Source: CAD feature listing. Evaluate the final solid. Frame: model axes, mm. A direction names the side the tool comes from. Give positions to 0.01 mm unless a question says otherwise; leave off trailing zeros. Order: outer loops, then holes, each group sorted by start corner. A loop starts at its lowest first (then second) coordinate and runs counter-clockwise, first axis right, second up. Notation, with made-up numbers: (45.5, 18) - (54.5, 18) arc R26 ccw to (54.5, 32) - close; hole circle Ø4 at (45.5, -11.5). An arc over 180 degrees is marked (long way). One line per item, written item: value. Start each with the question number.
Autodesk Inventor part; units mm, degrees
ref_plane "YZ Plane" through (0, 0, 0) normal (1, 0, 0) x (0, 1, 0)
ref_plane "XZ Plane" through (0, 0, 0) normal (0, 1, 0) x (-1, 0, 0)
ref_plane "XY Plane" through (0, 0, 0) normal (0, 0, 1) x (1, 0, 0)
sketch "Sketch1" plane through (0, 0, 0) normal (0, 1, 0) x (-1, 0, 0)
  line L0 (0, 4.9984) -> (-15, 4.9984)
  line L1 (-15, 4.9984) -> (-15, -15.0016)
  line L2 (-15, -15.0016) -> (0, -15.0016)
  line L3 (0, -15.0016) -> (0, 4.9984)
  dimension "d0" = 15
  dimension "d1" = 20
extrude "Plate1" add sketch "Sketch1" along normal blind 0.5
sketch "Sketch2" plane through (0, 1.3536, -15.3552) normal (0, 0.7071068, -0.7071068) x (-1, 0, 0)
  line L0 (-15, 0) -> (0, 0)
  line L1 (0, 0) -> (0, 2.5858)
  line L2 (0, 2.5858) -> (-15, 2.5858)
  line L3 (-15, 2.5858) -> (-15, 0)
edge flange "Flange1" height 5 angle 135 thickness 0.5 bend radius 0.5 thickness toward (0, 0.7071068, -0.7071068) relief tear relief width 0.5 relief depth 0.25 edges at (7.5, 0.5, -15.0016) wall of the first edge with corners at (15, 1.3536, -15.3552) (0, 1.3536, -15.3552) (0, 3.182, -13.5267) (15, 3.182, -13.5267)
bend "Bend1"
corner "Corner1"
sketch "Sketch3" plane through (15, 3.8891, -13.7338) normal (0, 0, 1) x (1, 0, 0)
  line L0 (-15, 0) -> (0, 0)
  line L1 (0, 0) -> (0, 26.5858)
  line L2 (0, 26.5858) -> (-15, 26.5858)
  line L3 (-15, 26.5858) -> (-15, 0)
edge flange "Flange2" height 27 angle 45 thickness 0.5 bend radius 0.5 thickness toward (0, 0, 1) relief tear relief width 0.5 relief depth 0.25 edges at (7.5, 3.5355, -13.8803) wall of the first edge with corners at (0, 3.8891, -13.7338) (15, 3.8891, -13.7338) (15, 30.4749, -13.7338) (0, 30.4749, -13.7338)
bend "Bend2"
corner "Corner2"
sketch "Sketch4" plane through (0, 0, 0) normal (0, -1, 0) x (1, 0, 0)
  circle A0 centre (10, 2.4984) radius 1
  circle A1 centre (5, 2.4984) radius 1
  circle A2 centre (5, -7.5016) radius 1
  circle A3 centre (10, -7.5016) radius 1
  point P0 (0, 0)
extrude "Extrusion1" cut sketch "Sketch4" against normal blind 10
equation "\"d2\" = Thickness"
equation "\"d3\" = BendReliefWidth"
equation "\"d4\" = BendReliefDepth"
equation "\"d5\" = MinimumRemnant"
equation "\"d6\" = TransitionRadius"
equation "\"d9\" = BendRadius"
equation "\"d10\" = CornerReliefSize"
equation "\"d11\" = GapSize"
equation "\"d12\" = JacobiRadiusSize"
equation "\"d13\" = BendReliefWidth"
equation "\"d14\" = BendReliefDepth"
equation "\"d15\" = MinimumRemnant"
equation "\"d16\" = TransitionRadius"
equation "\"d19\" = BendRadius"
equation "\"d20\" = CornerReliefSize"
equation "\"d21\" = GapSize"
equation "\"d22\" = JacobiRadiusSize"
equation "\"BendRadius\" = Thickness"
equation "\"BendReliefWidth\" = Thickness"
equation "\"BendReliefDepth\" = 0.5 * Thickness"
equation "\"CornerReliefSize\" = 4 * Thickness"
equation "\"MinimumRemnant\" = 2 * Thickness"
equation "\"TransitionRadius\" = BendRadius"
equation "\"JacobiRadiusSize\" = BendRadius"
equation "\"GapSize\" = Thickness"
properties part number "LaminaResorte" material "Stainless Steel"
1. Draft query along X for faces 5 (the cylindrical face through (4.2, 0.2, -8.1)), 6 (the cylindrical face through (7.4, 0.82, -15.47)). Return one class per face: pulls with the +X half, pulls with the -X half, needs draft (parallel to the pull), parting line crosses it, or undercut.
2. Section B-B on z = 3. Return the cut outline in (x, y), then the cut area to 3 significant figures.
3. Section D-D on y = 23.5. Return the cut outline in (x, z).
4. Contact query for flat-ended pins moving along their axis: pin 1 Ø2.5 at (x, z) = (5, -7.5) entering from +Y; pin 2 Ø4 at (y, z) = (15.5, -9.5) entering from -X; pin 3 Ø1 at (x, y) = (6, 8) entering from +Z; pin 4 Ø8 at (x, y) = (3.5, 26) entering from -Z. Output: stop coordinate, or through.
5. Section A-A on x = 10. Return the cut outline in (y, z).
6. Set-up query: faces 1 (the flat face through (8, 17, -13.734)), 2 (the flat face through (8, 17, -13.234)), 3 (the cylindrical face through (7, 1, -16)), 4 (the flat face through (7.395, 2.255, -14.454)). Return all of +Z, -Z, +X, -X, +Y, -Y with unobstructed straight access to the full face (end or side cutting, diameter ignored); none if empty.
7. Ray query, L1, parallel to Z at x = 5, y = 0.3; L2, parallel to Z at x = 10, y = 0.4; L3, parallel to Z at x = 6.5, y = 5. Return the intervals inside material, ascending.
8. Section C-C on x = 3. Return the cut outline in (y, z).
Data:
1. face 5: undercut
1. face 6: needs draft
2. outline: (0, 0) - (4.13, 0) - (4.13, 0.5) - (0, 0.5) - close; (5.87, 0) - (9.13, 0) - (9.13, 0.5) - (5.87, 0.5) - close; (10.87, 0) - (15, 0) - (15, 0.5) - (10.87, 0.5) - close
2. area: 5.77 mm2
3. outline: (0, -13.73) - (15, -13.73) - (15, -13.23) - (0, -13.23) - close
4. pin 1: stops at y = 0.5
4. pin 2: passes through
4. pin 3: stops at z = -13.23
4. pin 4: stops at z = -13.73
5. outline: (0, -15) arc R1 ccw to (1.71, -15.71) - (3.54, -13.88) arc R0.5 cw to (3.89, -13.73) - (30.47, -13.73) - (30.47, -13.23) - (3.89, -13.23) arc R1 ccw to (3.18, -13.53) - (1.35, -15.36) arc R0.5 cw to (0.5, -15) - (0.5, -8.5) - (0, -8.5) - close; (0, -6.5) - (0.5, -6.5) - (0.5, 1.5) - (0, 1.5) - close; (0, 3.5) - (0.5, 3.5) - (0.5, 5) - (0, 5) - close
6. face 1: -Z, +X, -X, +Y
6. face 2: +Z, +X, -X, +Y
6. face 3: -Z, +X, -X
6. face 4: +Z, +X, -X
7. L1: z = -15.72 to -8.5, -6.5 to 1.5, 3.5 to 5
7. L2: z = -15.8 to -8.5, -6.5 to 1.5, 3.5 to 5
7. L3: z = -13.73 to -13.23
8. outline: (0, -15) arc R1 ccw to (1.71, -15.71) - (3.54, -13.88) arc R0.5 cw to (3.89, -13.73) - (30.47, -13.73) - (30.47, -13.23) - (3.89, -13.23) arc R1 ccw to (3.18, -13.53) - (1.35, -15.36) arc R0.5 cw to (0.5, -15) - (0.5, 5) - (0, 5) - close
